Here's how the part is built. I have some questions about the finished solid (model axes, mm). Face numbers are marked on the shaded views. A direction names the side the tool comes from. Round coordinates to 2 decimals unless told otherwise and drop trailing zeros. Loops run counter-clockwise (first coordinate to the right, second up) from the corner with the lowest first, then second, coordinate; pieces in that order, holes last. Notation, with made-up numbers: M -25.5,9.25 L 27.5,9.25 A22 cw 27.5,35.25 Z; hole C 60.5,36 d6. An arc over 180 degrees is marked long. Answer as a JSON object with one key per item and string values.
Autodesk Inventor part; units mm, degrees
ref_plane "YZ Plane" through (0, 0, 0) normal (1, 0, 0) x (0, 1, 0)
ref_plane "XZ Plane" through (0, 0, 0) normal (0, 1, 0) x (-1, 0, 0)
ref_plane "XY Plane" through (0, 0, 0) normal (0, 0, 1) x (1, 0, 0)
sketch "Sketch1" plane through (0, 0, 0) normal (0, 0, 1) x (1, 0, 0)
  circle A0 centre (0, 0) radius 7.9
  dimension "d0" = 15.8
extrude "Extrusion1" add sketch "Sketch1" along normal blind 2
sketch "Sketch2" plane through (0, 0, 2) normal (0, 0, 1) x (1, 0, 0)
  circle A0 centre (0, 0) radius 7.9
  circle A1 centre (0, 0) radius 7.9
  circle A2 centre (0, 0) radius 6.05
  dimension "d4" = 12.1
extrude "Extrusion2" add sketch "Sketch2" along normal blind 3.8
sketch "Sketch3" plane through (0, 0, 2) normal (0, 0, 1) x (1, 0, 0)
  circle A0 centre (0, 0) radius 6.05
  circle A1 centre (0, 0) radius 3.5
  dimension "d8" = 7
extrude "Extrusion3" cut sketch "Sketch3" against normal blind 4 contours A1
properties part number "Bearring cap 8mm"
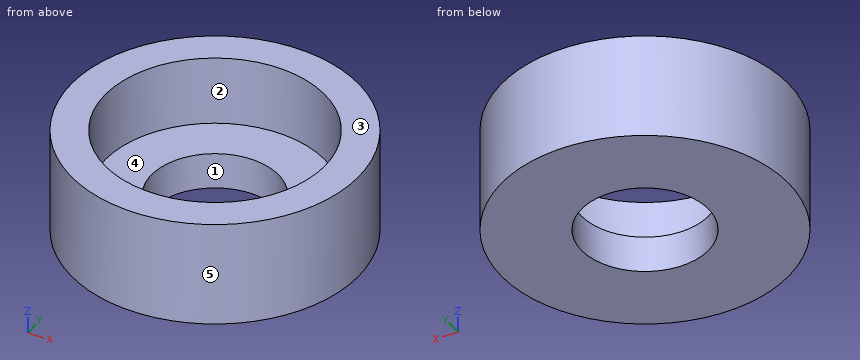
Item 1: For the marked faces 1 and 2, which set-ups out of +Z, -Z, +X, -X, +Y, -Y let a thin tool reach every point of the face, with its end or its side?
Solution:
{"face 1": "+Z, -Z", "face 2": "+Z"}
Item 2: If I drill on L1, parallel to Y at x = 0, z = 0.5; L2, parallel to Z at x = -5, y = -0.25; L3, parallel to Y at x = 0, z = 3.05, over which ranges is the centre line in solid material (lowest first)? Write a range as from..to.
Solution:
{"L1": "y = -7.9..-3.5, 3.5..7.9", "L2": "z = 0..2", "L3": "y = -7.9..-6.05, 6.05..7.9"}
Item 3: We'd pull the mould along X, two halves only. Please class the marked faces 3, 4 and 5: +X half, -X half, draft (parallel to the pull), parting line (faces both ways), or undercut.
Solution:
{"face 3": "draft", "face 4": "undercut", "face 5": "parting line"}
Item 4: For P1, Ø1.5, axis at x = -4.5, y = -2, coming from the +Z side; P2, Ø3.5, axis at x = 1, y = -1, coming from the +Z side; P3, Ø2, axis at y = -5.5, z = 2.5, coming from the +X side; P4, Ø1, axis at y = -3, z = 1.5, coming from the +X side, each with a flat end and sliding along its axis, tell me the tip position at first contact or that it passes through.
Solution:
{"P1": "stops at z = 2", "P2": "passes through", "P3": "stops at x = 6.49", "P4": "stops at x = 7.49"}
Item 5: I want a section at A-A on y = 0. List the corners of the cut face in (x, z) for me, plus the area to 3 significant figures.
Solution:
{"outline": "M -7.9,0 L -3.5,0 L -3.5,2 L -6.05,2 L -6.05,5.8 L -7.9,5.8 Z; M 3.5,0 L 7.9,0 L 7.9,5.8 L 6.05,5.8 L 6.05,2 L 3.5,2 Z", "area": "31.7 mm2"}
Item 6: I want a section at C-C on x = -5. List the corners of the cut face in (y, z) for me, plus the area to 3 significant figures.
Solution:
{"outline": "M -6.12,0 L 6.12,0 L 6.12,5.8 L 3.41,5.8 L 3.41,2 L -3.41,2 L -3.41,5.8 L -6.12,5.8 Z", "area": "45.1 mm2"}
Item 7: I want a section at D-D on z = 4. List the corners of the cut face in (x, y) for me.
Solution:
{"outline": "C 0,0 d15.8; hole C 0,0 d12.1"}
